Answer from the drawing. Dimensions are ordinates in mm from the lowest x, y and z of the part. Give positions to 0.01 mm unless a question says otherwise; leave off trailing zeros. Order: outer loops, then holes, each group sorted by start corner. A loop starts at its lowest first (then second) coordinate and runs counter-clockwise, first axis right, second up.
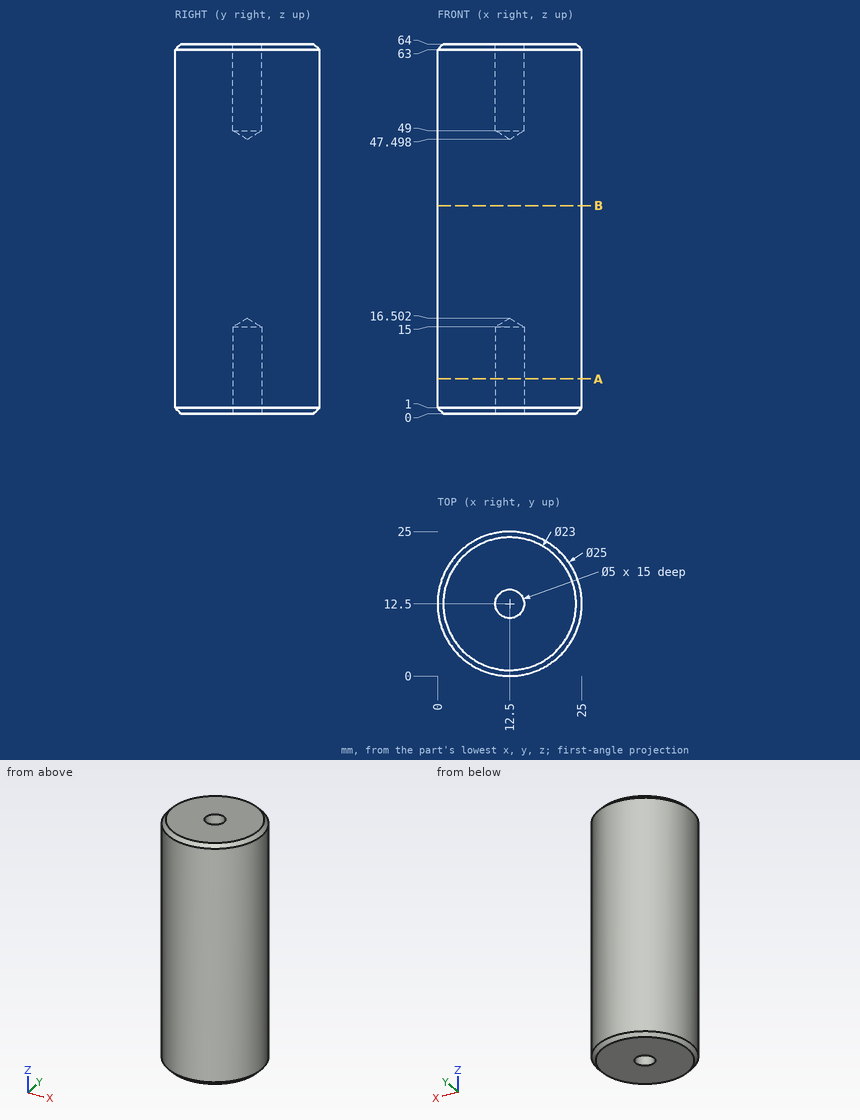
1) The part is cut by section A-A on z = 6. Determine the outline of the cut face in (x, y).
Final values:
outline: circle Ø25 at (12.5, 12.5); hole circle Ø5 at (12.5, 12.5)
2) The part is cut by section B-B on z = 36. Determine the outline of the cut face in (x, y), and give its area (3 significant figures).
Final values:
outline: circle Ø25 at (12.5, 12.5)
area: 491 mm2
3) Given pin 1 (4 mm diameter, centred on x = 12.5, y = 12.5, fed in from +Z); pin 2 (6 mm diameter, centred on x = 21, z = 54.5, fed in from +Y) (3 decimals); pin 3 (1.5 mm diameter, centred on y = 4.5, z = 10.5, fed in from -X), each flat-ended and moving along its own axis, determine where each tip first touches the part or whether it passes through.
Final values:
pin 1: stops at z = 48.7
pin 2: stops at y = 23.725
pin 3: stops at x = 2.32
4) Consider L1, parallel to Y at x = 12.5, z = 4.75; L2, parallel to Y at x = 4.25, z = 61.5; L3, parallel to Z at x = 2.75, y = 19.5. Determine where each line is inside the solid, lowest interval first.
Final values:
L1: y = 0 to 10, 15 to 25
L2: y = 3.11 to 21.89
L3: z = 0.5 to 63.5
